from build123d import *

# Parameters (mm, degrees)
SKETCH1_R          = 7.9375
SKETCH1_R_2        = 3.2004
EXTRUDE1_DEPTH     = 25.4
SKETCH5_R          = 7.9375
SKETCH5_R_2        = 3.2004
CUT_EXTRUDE1_DEPTH = 3.175
SKETCH6_R          = 4.7625
CUT_EXTRUDE2_DEPTH = 48.625


with BuildPart() as part:
    # Sketch1 → Extrude1 (new body, symmetric)
    with BuildSketch(Plane.XY):
        Circle(SKETCH1_R)
        Circle(SKETCH1_R_2, mode=Mode.SUBTRACT)
    extrude(amount=EXTRUDE1_DEPTH, both=True)

    # Sketch5 → Cut-Extrude1 (cut)
    with BuildSketch(Plane.XY.offset(25.4)):
        Circle(SKETCH5_R)
        Circle(SKETCH5_R_2, mode=Mode.SUBTRACT)
    extrude(amount=-CUT_EXTRUDE1_DEPTH, mode=Mode.SUBTRACT)

    # Sketch6 → Cut-Extrude2 (cut, through all)
    with BuildSketch(Plane.XY.offset(22.225)):
        Circle(SKETCH6_R)
    extrude(amount=-CUT_EXTRUDE2_DEPTH, mode=Mode.SUBTRACT)


solid = part.part
Geometry: final body of the model. Coordinates: model frame, mm. Give positions to 0.01 mm unless a question says otherwise; leave off trailing zeros. Write each loop counter-clockwise with the first axis right and the second up, starting at its lowest first coordinate (ties: lowest second). Pieces come first, ordered by that corner, then holes. Notation, with made-up numbers: M -14.75,-12 L 10.25,-12 A21 ccw 10.25,19 Z; hole C 38,7 d7. An arc over 180 degrees is marked long. Answer in a Markdown table with one row per item. Add a question column.
(1) Ray query, line 1 (Y direction, x = 0, z = 2.5); line 2 (Y direction, x = 2.5, z = 2.5); line 3 (X direction, y = -3.75, z = 7). Return the intervals inside material, ascending.
(2) Mould query, pull axis X, two halves, no side actions, for faces 1 (the cylindrical face through (-1.72, -7.75, -1.25)), 2 (the flat face through (0, -5, 22.225)), 3 (the cylindrical face through (-3.78, -2.9, -1.25)). Classes: +X half, -X half, draft (parallel to the pull), parting line (faces both ways), or undercut.
(3) Section A-A on x = 0. Return loops of the section in (y, z) (1 decimal).
(4) Section B-B on y = -2.75. Return loops of the section in (x, z) (3 decimals), and give its area (3 significant figures).
(5) First-contact query: pin 1 (4 mm diameter, centred on x = -1.5, y = -2, fed in from -Z); pin 2 (4 mm diameter, centred on x = 3, z = -17, fed in from -Y); pin 3 (1 mm diameter, centred on x = 5, z = 6, fed in from -Y); pin 4 (6 mm diameter, centred on x = 2, z = -10, fed in from +Y). Flat tips, straight axial feed; report the tip coordinate or a pass-through.
(6) Section C-C on z = 1. Return loops of the section in (x, y) (1 decimal), and give its area (3 significant figures).
(7) Section D-D on y = 6.75. Return loops of the section in (x, z) (3 decimals), and give its area (3 significant figures).
Result set:
| question | item | result |
|---|---|---|
| 1 | line 1 | y = -7.94 to -4.76, 4.76 to 7.94 |
| 1 | line 2 | y = -7.53 to -4.05, 4.05 to 7.53 |
| 1 | line 3 | x = -7 to -2.94, 2.94 to 7 |
| 2 | face 1 | parting line |
| 2 | face 2 | draft |
| 2 | face 3 | undercut |
| 3 | outline | M -7.9,-25.4 L -4.8,-25.4 L -4.8,22.2 L -7.9,22.2 Z; M 4.8,-25.4 L 7.9,-25.4 L 7.9,22.2 L 4.8,22.2 Z |
| 4 | outline | M -7.446,-25.4 L -3.888,-25.4 L -3.888,22.225 L -7.446,22.225 Z; M 3.888,-25.4 L 7.446,-25.4 L 7.446,22.225 L 3.888,22.225 Z |
| 4 | area | 339 mm^2 |
| 5 | pin 1 | passes through |
| 5 | pin 2 | stops at y = -7.87 |
| 5 | pin 3 | stops at y = -6.54 |
| 5 | pin 4 | stops at y = 7.94 |
| 6 | outline | C 0,0 d15.9; hole C 0,0 d9.5 |
| 6 | area | 127 mm^2 |
| 7 | outline | M -4.176,-25.4 L 4.176,-25.4 L 4.176,22.225 L -4.176,22.225 Z |
| 7 | area | 398 mm^2 |
